Design review of the part built by this model. Coordinates are the model's own, in mm. A direction names the side the tool comes from. Round coordinates to 2 decimals unless told otherwise and drop trailing zeros. Order: outer loops, then holes, each group sorted by start corner. A loop starts at its lowest first (then second) coordinate and runs counter-clockwise, first axis right, second up. Notation, with made-up numbers: (10, 87) - (60, 87) arc R30 ccw to (60, 116) - close; hole circle Ø3 at (65.25, 43). An arc over 180 degrees is marked (long way). Use CSV: the item, a comma, the result in double quotes. Start each with the question number.
from build123d import *

# Parameters (mm, degrees)
F0_W        = 13
F0_H        = 13
F1_DEPTH    = 6
F2_W        = 10
F2_H        = 10
F3_DEPTH    = 4.5
F4_W        = 10
F4_H        = 2
F5_DEPTH    = 12.5
F6_W        = 10
F6_H        = 2
F7_DEPTH    = 12.5
F8_T1_DEPTH = 2.285841494


# Not quite as in the source:
# - a fillet or chamfer that OpenCascade refuses, or shapes differently, is made with other operations: its cross-section is extruded or revolved along the edge and cut away or added


with BuildPart() as f1:
    # F0 (on Top) → F1 (new body)
    with BuildSketch(Plane.XY):
        Rectangle(F0_W, F0_H)
    extrude(amount=F1_DEPTH)

    # F2 (on Top) → F3 (cut)
    with BuildSketch(Plane.XY):
        Rectangle(F2_W, F2_H)
    extrude(amount=F3_DEPTH, mode=Mode.SUBTRACT)

    # F4 (on Right) → F5 (cut, symmetric)
    with BuildSketch(Plane.YZ):
        Rectangle(F4_W, F4_H)
    extrude(amount=F5_DEPTH, both=True, mode=Mode.SUBTRACT)

    # F6 (on Front) → F7 (cut, symmetric)
    with BuildSketch(Plane.XZ):
        Rectangle(F6_W, F6_H)
    extrude(amount=F7_DEPTH, both=True, mode=Mode.SUBTRACT)

    # F8: chamfer of 0.5 on 4 edges, made by hand

    # F8_s2 → F8_t1 (cut)
    with BuildSketch(Plane.XY.offset(-1.285841494)):
        Polygon((5.5, -5), (5, -5.5), (5, -5), align=None)
        Polygon((5, 5.5), (5.5, 5), (5, 5), align=None)
        Polygon((-5.5, -5), (-5, -5.5), (-5, -5), align=None)
        Polygon((-5, 5.5), (-5.5, 5), (-5, 5), align=None)
    extrude(amount=F8_T1_DEPTH, mode=Mode.SUBTRACT)


solid = f1.part
Q1. Tool access review of faces 1 (the flat face through (6, -5, 0.5)), 2 (the flat face through (0, 0, 4.5)), 3 (the flat face through (5, -6, 0.5)): name each direction out of +Z, -Z, +X, -X, +Y, -Y from which nothing blocks a thin tool from reaching the whole face with its end or side.
Q2. Take a section at B-B (y = 5.25). State the section outline as (x, z) points, plus the area to 3 significant figures.
Q3. Take a section at D-D (z = 1.9). State the section outline as (x, y) points, plus the area to 3 significant figures.
Q4. Take a section at A-A (z = 0.65). State the section outline as (x, y) points.
Q5. Clearance check with a flat-ended pin moving along its axis: pin 1 (3 mm diameter, centred on x = 0, y = -1.5, fed in from -Z). State where the tip first meets the part, or that it passes through.
Q6. The part is to be moulded in two halves that separate along X. For faces 4 (the flat face through (0, 5, 3)), 5 (the flat face through (0, 6.5, 4)), 6 (the flat face through (-6.5, 0, 4)), say which applies: +X half, -X half, draft (parallel to the pull), parting line (faces both ways), or undercut.
Q7. For L1, parallel to Y at x = 4.25, z = 3.95; L2, parallel to Z at x = -5.5, y = 0.75, list the stretches that pass through material, from the lowest coordinate up. Write a range as [from, to].
Findings below:
1,face 1,"-Z, +X, -X"
1,face 2,"-Z"
1,face 3,"-Z, +Y, -Y"
2,outline,"(-6.5, 0) - (-5.25, 0) - (-5.25, 1) - (5.25, 1) - (5.25, 0) - (6.5, 0) - (6.5, 6) - (-6.5, 6) - close"
2,area,"67.5 mm^2"
3,outline,"(-6.5, -6.5) - (6.5, -6.5) - (6.5, 6.5) - (-6.5, 6.5) - close; hole (-5, -5) - (5, -5) - (5, 5) - (-5, 5) - close"
3,area,"69.0 mm^2"
4,outline,"(-6.5, -6.5) - (-5, -6.5) - (-5, -5.5) - (-5.5, -5) - (-6.5, -5) - close; (-6.5, 5) - (-5.5, 5) - (-5, 5.5) - (-5, 6.5) - (-6.5, 6.5) - close; (5, -6.5) - (6.5, -6.5) - (6.5, -5) - (5.5, -5) - (5, -5.5) - close; (5, 5.5) - (5.5, 5) - (6.5, 5) - (6.5, 6.5) - (5, 6.5) - close"
5,pin 1,"stops at z = 4.5"
6,face 4,"undercut"
6,face 5,"draft"
6,face 6,"-X half"
7,L1,"y = [-6.5, -5], [5, 6.5]"
7,L2,"z = [1, 6]"
